Source: three-view drawing plus pictorial views. Frame: mm from the lowest corner of the part. A direction names the side the tool comes from. Coordinates: 2 decimals unless noted, no trailing zeros. Write each loop counter-clockwise with the first axis right and the second up, starting at its lowest first coordinate (ties: lowest second). Pieces come first, ordered by that corner, then holes. Notation, with made-up numbers: M 12.25,-10.75 L 56.25,-10.75 A18 cw 56.25,13.25 Z; hole C 22.25,-16 d2. An arc over 180 degrees is marked long. Use CSV: the item, a comma, the result in double quotes.
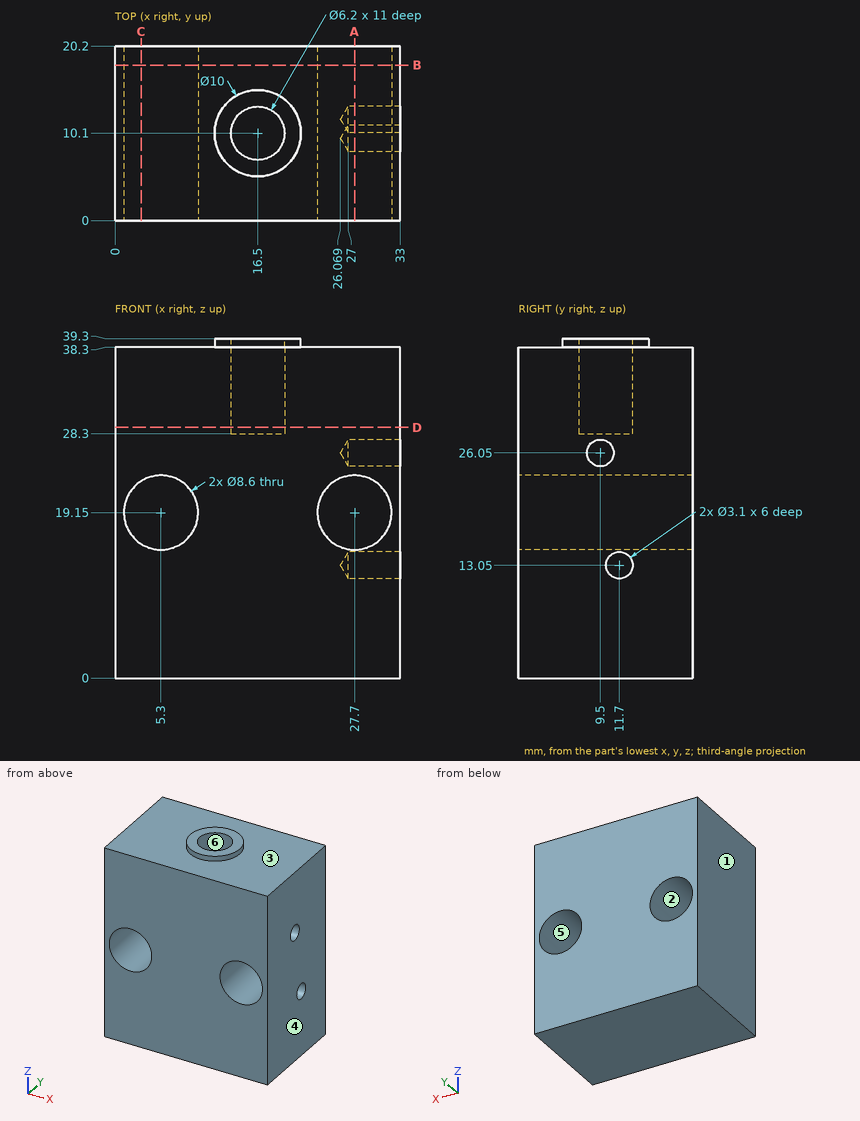
1. Contact query for flat-ended pins moving along their axis: pin 1 Ø3 at (x, y) = (16, 9.5) entering from +Z; pin 2 Ø5 at (x, z) = (5.3, 19.15) entering from -Y. Output: stop coordinate, or through.
Resolved:
pin 1,"stops at z = 28.3"
pin 2,"passes through"
2. Mould query, pull axis X, two halves, no side actions, for the marked faces 1, 2, 3 and 4. Classes: pulls with the +X half, pulls with the -X half, needs draft (parallel to the pull), parting line crosses it, or undercut.
Resolved:
face 1,"pulls with the -X half"
face 2,"undercut"
face 3,"needs draft"
face 4,"pulls with the +X half"
3. Material intervals for line 1 (Z direction, x = 31, y = 12) (1 decimal); line 2 (X direction, y = 6.75, z = 20.5); line 3 (X direction, y = 10, z = 37), sorted ascending. Write a range as [from, to].
Resolved:
line 1,"z = [0, 11.5], [14.6, 16.4], [21.9, 38.3]"
line 2,"x = [0, 1.22], [9.38, 23.62], [31.78, 33]"
line 3,"x = [0, 13.4], [19.6, 33]"
4. Section B-B (y = 18). Return loops of the section in (x, z), then the cut area to 3 significant figures.
Resolved:
outline,"M 0,0 L 33,0 L 33,38.3 L 0,38.3 Z; hole C 5.3,19.15 d8.6; hole C 27.7,19.15 d8.6"
area,"1,150 mm^2"
5. Section C-C (x = 3). Return loops of the section in (y, z), then the cut area to 3 significant figures.
Resolved:
outline,"M 0,0 L 20.2,0 L 20.2,15.52 L 0,15.52 Z; M 0,22.78 L 20.2,22.78 L 20.2,38.3 L 0,38.3 Z"
area,"627 mm^2"
6. Section D-D (z = 29). Return loops of the section in (x, y).
Resolved:
outline,"M 0,0 L 33,0 L 33,20.2 L 0,20.2 Z; hole C 16.5,10.1 d6.2"
7. Section A-A (x = 27.7). Return loops of the section in (y, z).
Resolved:
outline,"M 0,0 L 20.2,0 L 20.2,14.85 L 0,14.85 Z; M 0,23.45 L 20.2,23.45 L 20.2,38.3 L 0,38.3 Z; hole C 9.5,26.05 d3.1; hole C 11.7,13.05 d3.1"
8. Access query for the marked faces 5 and 6. Directions: +Z, -Z, +X, -X, +Y, -Y. A direction counts if a zero-diameter tool reaches every point of the face in a straight line with its end or side. Return the directions, or none.
Resolved:
face 5,"+Y, -Y"
face 6,"+Z"
